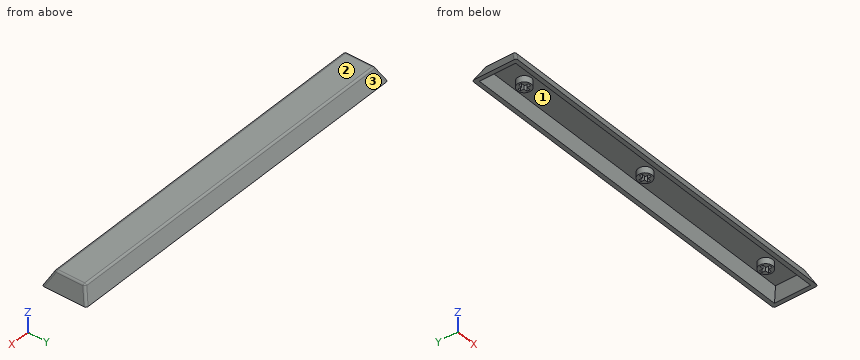
from build123d import *

# Parameters (mm, degrees)
F0_W        = 150
F0_H        = 18
F1_DEPTH    = 6
F2_T1_DEPTH = 49.0779464854
F2_T3_DEPTH = 181.0779464854
F3_R        = 1
F4_T        = -1.5
F5_R        = 2.8
F6_DEPTH    = 2.5
F7_W        = 1.5
F7_H        = 1.2
F7_W_2      = 1.2
F7_H_2      = 1.5
F8_DEPTH    = 2.5
F9_R        = 2.8
F10_DEPTH   = 2.5


# Not quite as in the source:
# - a fillet or chamfer that OpenCascade refuses, or shapes differently, is made with other operations: its cross-section is extruded or revolved along the edge and cut away or added


with BuildPart() as f1:
    # F0 (on Top) → F1 (new body)
    with BuildSketch(Plane.XY):
        Rectangle(F0_W, F0_H)
    extrude(amount=F1_DEPTH)

    # F2: chamfer of 3 x 6 on 4 edges, made by hand

    # F2_s2 → F2_t1 (cut)
    with BuildSketch(Plane.XZ.offset(-24.5389732427)):
        Polygon((75, 0), (72, 6), (75, 6), align=None)
        Polygon((-75, 0), (-72, 6), (-75, 6), align=None)
    extrude(amount=F2_T1_DEPTH, mode=Mode.SUBTRACT)

    # F2_s4 → F2_t3 (cut)
    with BuildSketch(Plane.YZ.offset(-90.5389732427)):
        Polygon((9, 0), (6, 6), (9, 6), align=None)
        Polygon((-9, 0), (-6, 6), (-9, 6), align=None)
    extrude(amount=F2_T3_DEPTH, mode=Mode.SUBTRACT)

    # F3
    f3_edges = [f1.edges().sort_by_distance(p)[0] for p in [
        (-73.5, 7.5, 3),
        (-73.5, -7.5, 3),
        (-72, 0, 6),
        (0, 6, 6),
        (72, 0, 6),
        (0, -6, 6),
        (73.5, 7.5, 3),
        (73.5, -7.5, 3),
    ]]
    fillet(f3_edges, radius=F3_R)

    # F4
    f4_openings = [f1.faces().sort_by_distance(p)[0] for p in [
        (0, 0, 0),
    ]]
    offset(amount=F4_T, openings=f4_openings)

    # F5 (on face) → F6 (join)
    with BuildSketch(Plane(origin=(0, 0, 4.5), x_dir=(1, 0, 0), z_dir=(0, 0, -1))):
        Circle(F5_R)
    extrude(amount=F6_DEPTH)

    # F7 (on face) → F8 (cut)
    with BuildSketch(Plane(origin=(0, 0, 2), x_dir=(1, 0, 0), z_dir=(0, 0, -1))):
        with Locations((-1.35, 0)):
            Rectangle(F7_W, F7_H)
        Rectangle(F7_W_2, F7_H)
        with Locations((0, -1.35)):
            Rectangle(F7_W_2, F7_H_2)
        with Locations((1.35, 0)):
            Rectangle(F7_W, F7_H)
        with Locations((0, 1.35)):
            Rectangle(F7_W_2, F7_H_2)
    extrude(amount=-F8_DEPTH, mode=Mode.SUBTRACT)

    # F9 (on face) → F10 (join)
    with BuildSketch(Plane(origin=(0, 0, 4.5), x_dir=(1, 0, 0), z_dir=(0, 0, -1))):
        with BuildLine():
            ThreePointArc((62.8, 0), (60, 2.8), (57.2, 0))
            ThreePointArc((57.2, 0), (60, -2.8), (62.8, 0))
        make_face()
        Polygon((57.9, -0.6), (57.9, 0), (57.9, 0.6), (59.4, 0.6), (59.4, 2.1), (60.6, 2.1), (60.6, 0.6), (62.1, 0.6), (62.1, -0.6), (60.6, -0.6), (60.6, -2.1), (59.4, -2.1), (59.4, -0.6), align=None, mode=Mode.SUBTRACT)
        with Locations((-60, 0)):
            Circle(F9_R)
        Polygon((-59.4, -0.6), (-59.4, -2.1), (-60.6, -2.1), (-60.6, -0.6), (-62.1, -0.6), (-62.1, 0.6), (-60.6, 0.6), (-60.6, 2.1), (-59.4, 2.1), (-59.4, 0.6), (-57.9, 0.6), (-57.9, -0.6), align=None, mode=Mode.SUBTRACT)
    extrude(amount=F10_DEPTH)


solid = f1.part
Here's how the part is built. I have some questions about the finished solid (model axes, mm). Face numbers are marked on the shaded views. Give positions to 0.01 mm unless a question says otherwise; leave off trailing zeros. Loops run counter-clockwise (first coordinate to the right, second up) from the corner with the lowest first, then second, coordinate; pieces in that order, holes last. Notation, with made-up numbers: (12, 3.25) -> (17, 3.25) arc R13 ccw to (17, 11.25) -> close; hole circle Ø2 at (62, 13.5). An arc over 180 degrees is marked (long way). Answer as a JSON object with one key per item and string values. Group by question number.
Item 1: I need wall thicknesses on L1, parallel to X at y = 6.75, z = 3.25; L2, parallel to Y at x = -63, z = 2.25 (3 decimals); L3, parallel to Z at x = 45, y = 5. Which ranges of each line are inside material? Lowest first, please.
Item 2: Thinking about a two-plate mould opening in Y: for the marked faces 1, 2 and 3, which applies, pulls with the +Y half, pulls with the -Y half, needs draft (parallel to the pull), parting line crosses it, or undercut?
Item 3: Will these pins go through, and if not, where does the flat tip stop? pin 1 (1.5 mm diameter, centred on y = 1.5, z = 1.5, fed in from -X) (3 decimals); pin 2 (1 mm diameter, centred on x = -18.5, z = 3, fed in from -Y); pin 3 (1 mm diameter, centred on y = 0.5, z = 3.5, fed in from -X).
Item 4: Imagine slicing it at A-A on x = 40. Write out the boundary of the cut face in (y, z), then the cut area to 3 significant figures.
Item 5: Imagine slicing it at B-B on z = 3.25. Give the number of separate pieces and of enclosed holes in the cut face, then the cut area to 3 significant figures.
Answer list:
{
 "1": {"L1": "x = -73.34 to 73.34", "L2": "y = -7.875 to -6.198, 6.198 to 7.875", "L3": "z = 4.5 to 6"},
 "2": {"face 1": "undercut", "face 2": "needs draft", "face 3": "pulls with the +Y half"},
 "3": {"pin 1": "stops at x = -74.625", "pin 2": "stops at y = -7.75", "pin 3": "stops at x = -73.5"},
 "4": {"outline": "(-9, 0) -> (-7.32, 0) -> (-5.07, 4.5) -> (5.07, 4.5) -> (7.32, 0) -> (9, 0) -> (6.28, 5.45) arc R1 ccw to (5.38, 6) -> (-5.38, 6) arc R1 ccw to (-6.28, 5.45) -> close", "area": "34.1 mm2"},
 "5": {"separate pieces": "4", "enclosed holes": "4", "area": "578 mm2"}
}
